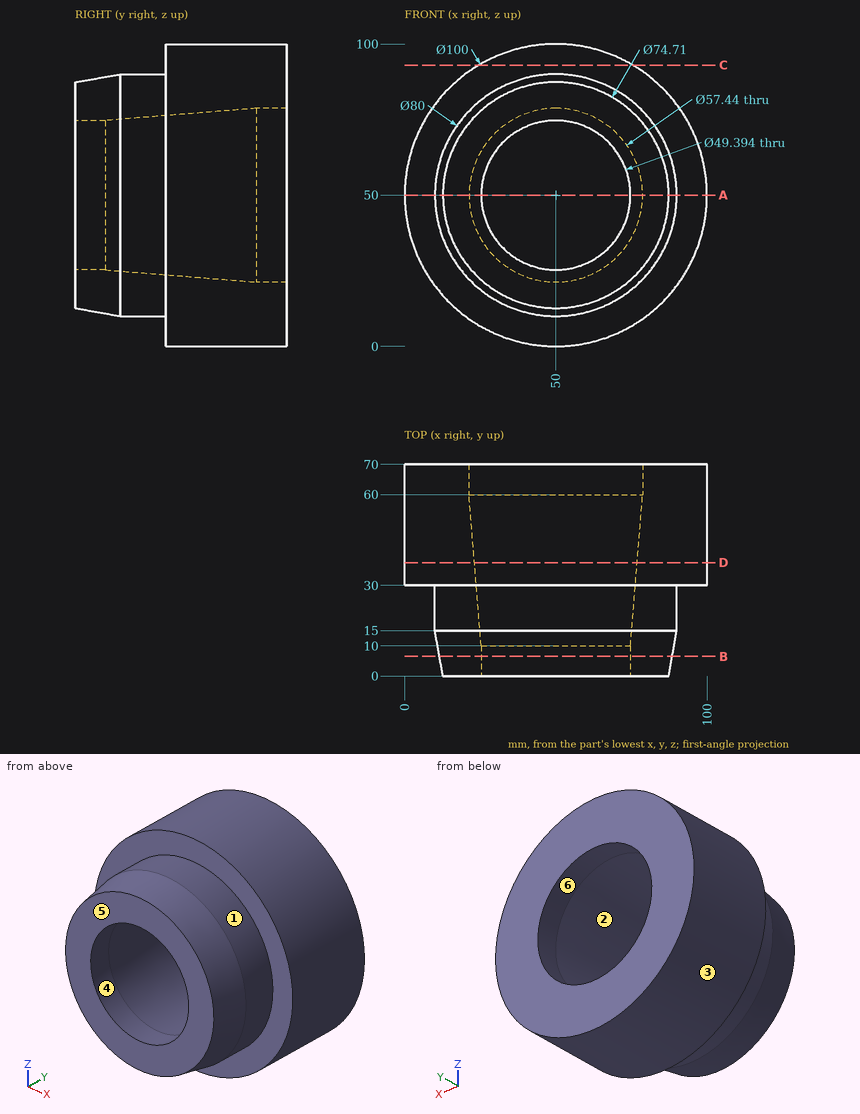
For this review, use the dimensioned drawing (mm, ordinates from the lowest corner) and the shaded views. A direction names the side the tool comes from. Give positions to 0.01 mm unless a question says otherwise; leave off trailing zeros. Write each loop counter-clockwise with the first axis right and the second up, starting at its lowest first coordinate (ties: lowest second). Pieces come first, ordered by that corner, then holes. Notation, with made-up numbers: M 6.25,51.5 L 27.25,51.5 A27 cw 27.25,73.5 Z; hole C 56.25,85.5 d5. An arc over 180 degrees is marked long. Answer as a JSON object with one key per item and string values. Group by question number.
1) For line 1 along Z through (x, y) = (50.5, 65); line 2 along Z through (x, y) = (74.5, 66.5) (1 decimal); line 3 along X through (y, z) = (4.25, 50) (1 decimal), list the stretches that pass through material, from the lowest coordinate up.
2) Clearance check with flat-ended pins moving along their axes: pin 1 Ø8 at (y, z) = (24.5, 37) entering from -X; pin 2 Ø1.5 at (x, y) = (22, 54.5) entering from +Z; pin 3 Ø2 at (x, y) = (38.5, 33.5) entering from +Z (3 decimals). State where each tip first meets the part, or that it passes through.
3) We need section D-D (y = 37.5). Give the boundary of the cut face in (x, z), and give its area (3 significant figures).
4) We need section A-A (z = 50). Give the boundary of the cut face in (x, y) (3 decimals), and give its area (3 significant figures).
5) Tool access review of the marked faces 1 and 2: name each direction out of +Z, -Z, +X, -X, +Y, -Y from which nothing blocks a thin tool from reaching the whole face with its end or side.
6) We need section B-B (y = 6.5). Give the boundary of the cut face in (x, z).
7) Mouldability with a two-part tool opening along Z and no side actions: class the marked faces 3, 4, 5 and 6 as released by +Z, released by -Z, zero draft, split by the parting line, or undercut.
8) We need section C-C (z = 93). Give the boundary of the cut face in (x, y) (1 decimal).
Answer key:
{
 "1": {"line 1": "z = 0 to 21.28, 78.72 to 100", "line 2": "z = 6.4 to 35, 65 to 93.6", "line 3": "x = 11.9 to 25.3, 74.7 to 88.1"},
 "2": {"pin 1": "stops at x = 11.03", "pin 2": "stops at z = 91.92", "pin 3": "stops at z = 98.885"},
 "3": {"outline": "C 50,50 d100; hole C 50,50 d53.82", "area": "5,580 mm²"},
 "4": {"outline": "M 0,30 L 10,30 L 10,15 L 12.645,0 L 25.303,0 L 25.303,10 L 21.28,60 L 21.28,70 L 0,70 Z; M 74.697,0 L 87.355,0 L 90,15 L 90,30 L 100,30 L 100,70 L 78.72,70 L 78.72,60 L 74.697,10 Z", "area": "2,620 mm²"},
 "5": {"face 1": "-Y", "face 2": "+Y"},
 "6": {"outline": "C 50,50 d77; hole C 50,50 d49.39"},
 "7": {"face 3": "split by the parting line", "face 4": "undercut", "face 5": "zero draft", "face 6": "undercut"},
 "8": {"outline": "M 24.5,30 L 75.5,30 L 75.5,70 L 24.5,70 Z"}
}
